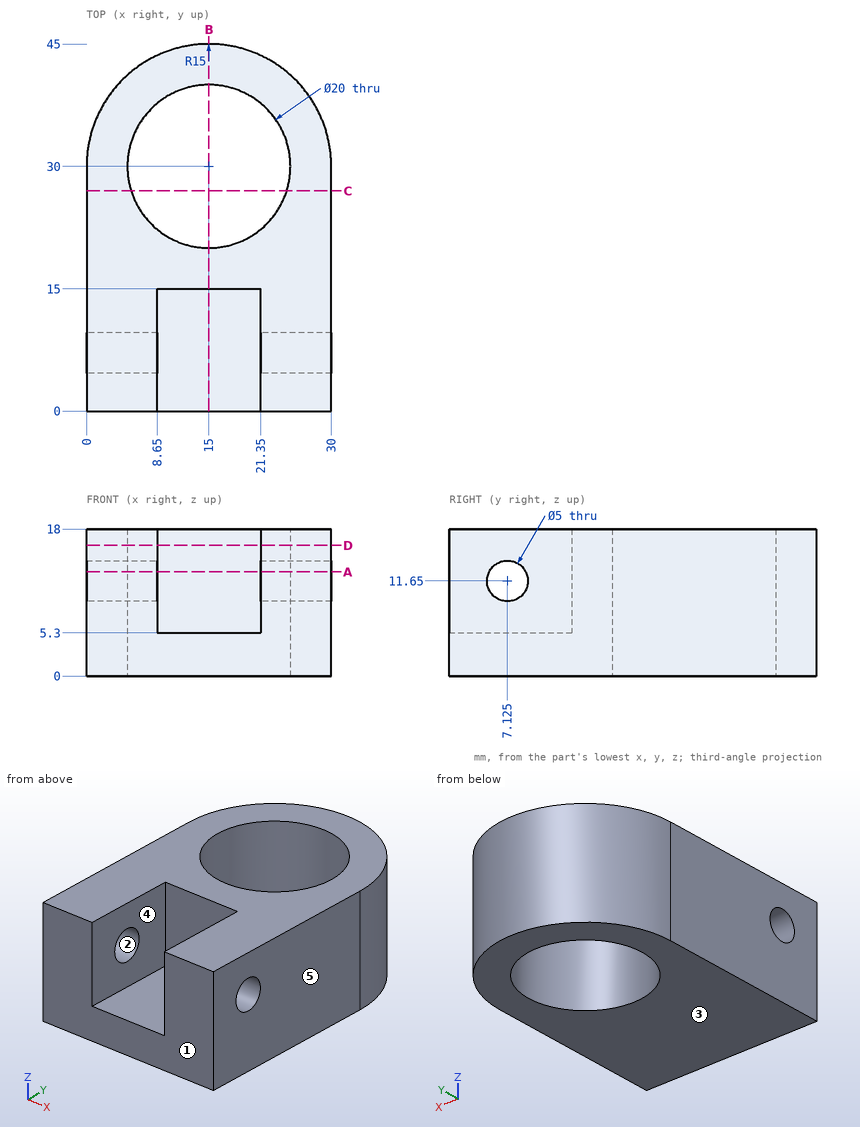
Study the drawing (mm; zero at the part's minimum x, y, z) and answer. A direction names the side the tool comes from. Coordinates: 2 decimals unless noted, no trailing zeros. Loops run counter-clockwise (first coordinate to the right, second up) from the corner with the lowest first, then second, coordinate; pieces in that order, holes last. Notation, with made-up numbers: M 56.5,6 L 70.5,6 A10 ccw 70.5,18 Z; hole C -32.75,-17 d2. An arc over 180 degrees is marked long. Answer in a Markdown table with one row per item. Add a question column.
1. The mould has two halves that part along Z. Classify the marked faces 1, 2 and 3: pulls with the +Z half, pulls with the -Z half, needs draft (parallel to the pull), parting line crosses it, or undercut.
2. Flat-ended cylindrical pins translate along their axes: P1, Ø4, axis at x = 4.5, z = 14.5, coming from the +Y side; P2, Ø18, axis at x = 15, y = 30, coming from the -Z side. Find the tip coordinate at first contact, or state that the pin passes through.
3. A tool of negligible diameter and unlimited length cuts with its end or side. For the marked faces 4 and 5, from which of +Z, -Z, +X, -X, +Y, -Y can it reach the whole face along a straight path? Write none if from no direction.
4. Find section D-D, the plane z = 16. Write down the section's boundary in (x, y).
5. Find section B-B, the plane x = 15. Write down the section's boundary in (y, z), then the cut area to 4 significant figures.
6. Consider L1, parallel to Y at x = 15, z = 6.5; L2, parallel to Y at x = 23.75, z = 11.65 (1 decimal); L3, parallel to Y at x = 26, z = 11.65 (3 decimals). Determine where each line is inside the solid, lowest interval first.
7. Find section A-A, the plane z = 12.75. Write down the section's boundary in (x, y), then the cut area to 3 significant figures.
8. Find section C-C, the plane y = 27. Write down the section's boundary in (x, z), then the cut area to 3 significant figures.
Reported:
| question | item | result |
|---|---|---|
| 1 | face 1 | needs draft |
| 1 | face 2 | undercut |
| 1 | face 3 | pulls with the -Z half |
| 2 | P1 | stops at y = 42.36 |
| 2 | P2 | passes through |
| 3 | face 4 | +Z, -Y |
| 3 | face 5 | +Z, -Z, +X, +Y, -Y |
| 4 | outline | M 0,0 L 8.65,0 L 8.65,15 L 21.35,15 L 21.35,0 L 30,0 L 30,30 A15 ccw 0,30 Z; hole C 15,30 d20 |
| 5 | outline | M 0,0 L 20,0 L 20,18 L 15,18 L 15,5.3 L 0,5.3 Z; M 40,0 L 45,0 L 45,18 L 40,18 Z |
| 5 | area | 259.5 mm^2 |
| 6 | L1 | y = 15 to 20, 40 to 45 |
| 6 | L2 | y = 0 to 4.6, 9.6 to 25.2, 34.8 to 42.2 |
| 6 | L3 | y = 0 to 4.625, 9.625 to 40.198 |
| 7 | outline | M 0,0 L 8.65,0 L 8.65,4.88 L 0,4.88 Z; M 0,9.37 L 8.65,9.37 L 8.65,15 L 21.35,15 L 21.35,9.37 L 30,9.37 L 30,30 A15 ccw 0,30 Z; M 21.35,0 L 30,0 L 30,4.88 L 21.35,4.88 Z; hole C 15,30 d20 |
| 7 | area | 671 mm^2 |
| 8 | outline | M 0,0 L 5.46,0 L 5.46,18 L 0,18 Z; M 24.54,0 L 30,0 L 30,18 L 24.54,18 Z |
| 8 | area | 197 mm^2 |
